Model file for the job. Use its own axes, mm. A direction names the side the tool comes from. Coordinates: 2 decimals unless noted, no trailing zeros. Write each loop counter-clockwise with the first axis right and the second up, starting at its lowest first coordinate (ties: lowest second). Pieces come first, ordered by that corner, then holes. Notation, with made-up numbers: (17.5, 66.5) -> (56.5, 66.5) arc R20 cw to (56.5, 86.5) -> close; hole circle Ø11 at (18, 73.25). An arc over 180 degrees is marked (long way). Answer as a JSON object with one key per item and string values. Group by question number.
from build123d import *

# Parameters (mm, degrees)
ESBO_O1_R                = 1.5
RESSALTO_EXTRUS_O1_DEPTH = 5
RESSALTO_EXTRUS_O2_START = 8
ESBO_O2_R                = 5
RESSALTO_EXTRUS_O2_DEPTH = 8
ESBO_O3_R                = 10
RESSALTO_EXTRUS_O3_DEPTH = 5


with BuildPart() as part:
    # Esboço1 → Ressalto-extrusão1 (new body)
    with BuildSketch(Plane.YZ):
        with BuildLine():
            Line((5, 42.5), (5, -117.8))
            ThreePointArc((5, -117.8), (0, -122.8), (-5, -117.8))
            Line((-5, -117.8), (-5, 42.5))
            ThreePointArc((-5, 42.5), (0, 47.5), (5, 42.5))
        make_face()
        with Locations(Location((0, 0, 0), (0, 0, 270))):
            Circle(ESBO_O1_R, mode=Mode.SUBTRACT)
    extrude(amount=RESSALTO_EXTRUS_O1_DEPTH)

    # Esboço2 → Ressalto-extrusão2 (add)
    with BuildSketch(Plane(origin=(0, 0, 0), x_dir=(0, -1, 0), z_dir=(-1, 0, 0)).offset(RESSALTO_EXTRUS_O2_START)):
        with Locations(Location((0, 42.5, 0), (0, 0, 90))):
            Circle(ESBO_O2_R)
    extrude(amount=-RESSALTO_EXTRUS_O2_DEPTH)

    # Esboço3 → Ressalto-extrusão3 (add)
    with BuildSketch(Plane(origin=(0, 0, 0), x_dir=(0, -1, 0), z_dir=(-1, 0, 0))):
        with Locations((0, -117.8)):
            Circle(ESBO_O3_R)
    extrude(amount=-RESSALTO_EXTRUS_O3_DEPTH)


solid = part.part
(1) Pull direction Y, two halves, no side cores. Call faces 1 (the face through (2.465, 0.366, -127.793)), 2 (the face through (-8, 0, 42)), 3 (the face through (2.46, 0.45, -1.43)), 4 (the face through (2, 5, -32)): released by +Y, released by -Y, zero draft, split by the parting line, or undercut.
(2) Cut at A-A on z = 0. List the corners of the cut face in (x, y), plus the area to 3 significant figures.
(3) Cut at C-C on z = -35. List the corners of the cut face in (x, y), plus the area to 3 significant figures.
(4) Cut at D-D on x = -5.25. List the corners of the cut face in (y, z), plus the area to 3 significant figures.
(5) Cut at B-B on y = -8. List the corners of the cut face in (x, z), plus the area to 3 significant figures.
(6) 3-axis set-ups, long thin cutter, end or side, ignore diameter. For faces 5 (the face through (2, -5, -34)), 6 (the face through (5, 0, -39)): which of +Z, -Z, +X, -X, +Y, -Y reach the whole face in a straight line?
(7) Wall check: probe 1 along Y at (x, z) = (1.9, 0); probe 2 along X at (y, z) = (-3, -113); probe 3 along Z at (x, y) = (-6.25, 0.5). Give the ranges that are in metal, low to high.
(8) Pin check, flat tips, straight feed: pin 1 (2.5 mm diameter, centred on x = 2.5, z = -6, fed in from +Y); pin 2 (2 mm diameter, centred on x = 3, y = 1.5, fed in from -Z); pin 3 (2 mm diameter, centred on y = -3, z = -22, fed in from -X); pin 4 (3.5 mm diameter, centred on y = 0, z = 0, fed in from +X). Stop position of each tip, or through.
Results found:
{
 "1": {"face 1": "split by the parting line", "face 2": "zero draft", "face 3": "undercut", "face 4": "released by +Y"},
 "2": {"outline": "(0, -5) -> (5, -5) -> (5, -1.5) -> (0, -1.5) -> close; (0, 1.5) -> (5, 1.5) -> (5, 5) -> (0, 5) -> close", "area": "35.0 mm²"},
 "3": {"outline": "(0, -5) -> (5, -5) -> (5, 5) -> (0, 5) -> close", "area": "50.0 mm²"},
 "4": {"outline": "circle Ø10 at (0, 42.5)", "area": "78.5 mm²"},
 "5": {"outline": "(0, -123.8) -> (5, -123.8) -> (5, -111.8) -> (0, -111.8) -> close", "area": "60.0 mm²"},
 "6": {"face 5": "+Z, +X, -X, -Y", "face 6": "+Z, -Z, +X, +Y, -Y"},
 "7": {"probe 1": "y = -5 to -1.5, 1.5 to 5", "probe 2": "x = 0 to 5", "probe 3": "z = 37.53 to 47.47"},
 "8": {"pin 1": "stops at y = 5", "pin 2": "stops at z = -127.79", "pin 3": "stops at x = 0", "pin 4": "stops at x = 5"}
}
